Can you work these out from the model? Positions are in its coordinate system, mm. Face numbers are marked on the shaded views. Round coordinates to 2 decimals unless told otherwise and drop trailing zeros. Loops run counter-clockwise (first coordinate to the right, second up) from the corner with the lowest first, then second, coordinate; pieces in that order, holes last. Notation, with made-up numbers: M -7,25 L 12,25 A23 ccw 12,60 Z; hole C 53,-17.5 d3. An arc over 180 degrees is marked long. Answer as CSV lines item,"result".
from build123d import *

# Parameters (mm, degrees)
F0_R      = 15
F0_R_2    = 13
F1_DEPTH  = 100
F3_R      = 25
F3_R_2    = 15
F4_DEPTH  = 4
F5_R      = 2
F6_DEPTH  = 96.001
F7_R      = 18.5
F7_R_2    = 13
F8_DEPTH  = 15
F9_R      = 2
F10_DEPTH = 50
F11_R     = 2
F12_DEPTH = 50
F13_SIZE  = 2.99999
F14_SIZE  = 3
F15_R     = 14
F16_DEPTH = 20
F17_R     = 2
F18_DEPTH = 25
F19_R     = 1.5
F20_DEPTH = 6


# Not quite as in the source:
# - a fillet or chamfer is up to 0.001 mm smaller than in the source, because OpenCascade refuses the exact size


with BuildPart() as f1:
    # F0 (on Top) → F1 (new body)
    with BuildSketch(Plane.XY):
        Circle(F0_R)
        Circle(F0_R_2, mode=Mode.SUBTRACT)
    extrude(amount=F1_DEPTH)

    # F3 (on offset) → F4 (join)
    with BuildSketch(Plane.XY.offset(96)):
        Circle(F3_R)
        Circle(F3_R_2, mode=Mode.SUBTRACT)
    extrude(amount=-F4_DEPTH)

    # F5 (on face) → F6 (cut, through all)
    with BuildSketch(Plane.XY.offset(96)):
        with Locations((0, 20)):
            Circle(F5_R)
        with Locations((-20, 0)):
            Circle(F5_R)
        with Locations((0, -20)):
            Circle(F5_R)
        with Locations((20, 0)):
            Circle(F5_R)
    extrude(amount=-F6_DEPTH, mode=Mode.SUBTRACT)

    # F7 (on Top) → F8 (join)
    with BuildSketch(Plane.XY):
        Circle(F7_R)
        Circle(F7_R_2, mode=Mode.SUBTRACT)
    extrude(amount=F8_DEPTH)

    # F9 (on Right) → F10 (cut, symmetric)
    with BuildSketch(Plane.YZ):
        with Locations((0, 7.5)):
            Circle(F9_R)
    extrude(amount=F10_DEPTH, both=True, mode=Mode.SUBTRACT)

    # F11 (on Front) → F12 (cut, symmetric)
    with BuildSketch(Plane.XZ):
        with Locations((0, 7.5)):
            Circle(F11_R)
    extrude(amount=F12_DEPTH, both=True, mode=Mode.SUBTRACT)

    # F13 (size 3 in the source; OpenCascade refuses exactly that, so slightly less here)
    f13_edges = [f1.edges().sort_by_distance(p)[0] for p in [
        (-15, 0, 92),
    ]]
    chamfer(f13_edges, length=F13_SIZE)

    # F14
    f14_edges = [f1.edges().sort_by_distance(p)[0] for p in [
        (-15, 0, 15),
    ]]
    chamfer(f14_edges, length=F14_SIZE)

    # F15 (on face) → F16 (cut)
    with BuildSketch(Plane(origin=(0, 0, 0), x_dir=(1, 0, 0), z_dir=(0, 0, -1))):
        Circle(F15_R)
    extrude(amount=-F16_DEPTH, mode=Mode.SUBTRACT)

    # F17 (on face) → F18 (cut)
    with BuildSketch(Plane.XY.offset(96)):
        with Locations((14.1421356237, 14.1421356237)):
            Circle(F17_R)
    extrude(amount=-F18_DEPTH, mode=Mode.SUBTRACT)

    # F19 (on face) → F20 (cut)
    with BuildSketch(Plane(origin=(0, 0, 0), x_dir=(1, 0, 0), z_dir=(0, 0, -1))):
        with Locations((11.4904851943, -11.4904851943)):
            Circle(F19_R)
    extrude(amount=-F20_DEPTH, mode=Mode.SUBTRACT)


solid = f1.part
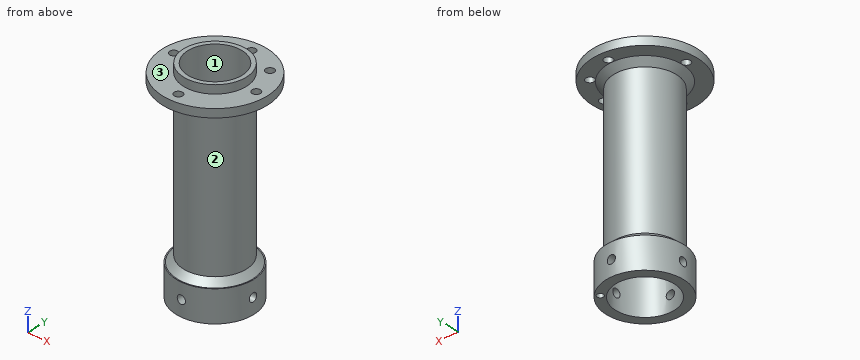
Item 1: If we section it at D-D on x = 0: State how many separate pieces and enclosed holes the cut face has, then the cut area to 3 significant figures.
Output:
separate pieces,"6"
enclosed holes,"0"
area,"495 mm2"
Item 2: Will these pins go through, and if not, where does the flat tip stop? pin 1 (4.5 mm diameter, centred on x = 14.14, y = 14.14, fed in from +Z); pin 2 (5 mm diameter, centred on x = -5.5, z = 60.5, fed in from +Y); pin 3 (4 mm diameter, centred on y = -11.5, z = 71.5, fed in from -X); pin 4 (3.5 mm diameter, centred on x = 0, z = 7.5, fed in from -Y).
Output:
pin 1,"stops at z = 96"
pin 2,"stops at y = 14.7"
pin 3,"stops at x = -11.61"
pin 4,"passes through"
Item 3: We'd pull the mould along Z, two halves only. Please class the marked faces 1, 2 and 3: released by +Z, released by -Z, zero draft, split by the parting line, or undercut.
Output:
face 1,"zero draft"
face 2,"undercut"
face 3,"released by +Z"
Item 4: If I drill on line 1 along Y through (x, z) = (0, 83); line 2 along Y through (x, z) = (0, 94); line 3 along Y through (x, z) = (-20, 95), over which ranges is the centre line in solid material (lowest first)? Write a range as from..to.
Output:
line 1,"y = -15..-13, 13..15"
line 2,"y = -25..-22, -18..-13, 13..18, 22..25"
line 3,"y = -15..-2, 2..15"
Item 5: If we section it at A-A on x = 20: Write out the boundary of the cut face in (y, z).
Output:
outline,"M -15,92 L -2,92 L -2,96 L -15,96 Z; M 2,92 L 15,92 L 15,96 L 2,96 Z"
Item 6: If we section it at C-C on z = 7.5: Write out the boundary of the cut face in (x, y).
Output:
outline,"M -18.39,-2 A18.5 ccw -2,-18.39 L -2,-13.86 A14 cw -13.86,-2 Z; M -18.39,2 L -13.86,2 A14 cw -2,13.86 L -2,18.39 A18.5 ccw Z; M 2,-18.39 A18.5 ccw 18.39,-2 L 13.86,-2 A14 cw 2,-13.86 Z; M 2,13.86 A14 cw 13.86,2 L 18.39,2 A18.5 ccw 2,18.39 Z"
